The drawing under review shows one solid part. Ordinate dimensions are in mm from its lowest x, y, z. Coordinates: 2 decimals unless noted, no trailing zeros. Write each loop counter-clockwise with the first axis right and the second up, starting at its lowest first coordinate (ties: lowest second). Pieces come first, ordered by that corner, then holes.
Q1. Add section A-A, the plane x = 15. Give the boundary of the cut face in (y, z) (3 decimals), plus the area to 3 significant figures.
Q2. Add section B-B, the plane y = 0.9. Give the number of separate pieces and of enclosed holes in the cut face, plus the area to 3 significant figures.
Q3. To check wall thickness, follow probe 1 along Z at (x, y) = (25, 1.15). State the ranges of the line that lie inside material, in increasing order.
Q4. Add section D-D, the plane x = 25.5. Give the boundary of the cut face in (y, z) (3 decimals), plus the area to 3 significant figures.
Q5. Add section C-C, the plane z = 25. Give the boundary of the cut face in (x, y) (3 decimals).
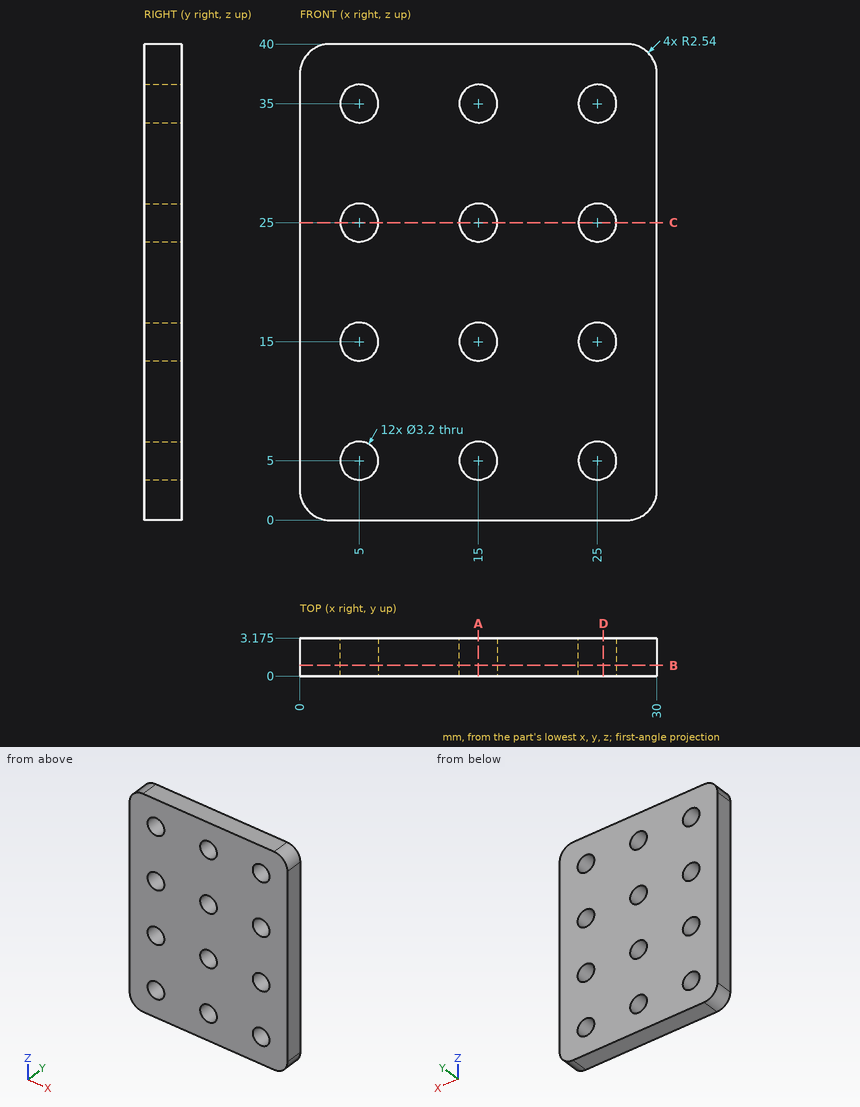
Here are the results:
1. outline: (0, 0) - (3.175, 0) - (3.175, 3.4) - (0, 3.4) - close; (0, 6.6) - (3.175, 6.6) - (3.175, 13.4) - (0, 13.4) - close; (0, 16.6) - (3.175, 16.6) - (3.175, 23.4) - (0, 23.4) - close; (0, 26.6) - (3.175, 26.6) - (3.175, 33.4) - (0, 33.4) - close; (0, 36.6) - (3.175, 36.6) - (3.175, 40) - (0, 40) - close
1. area: 86.4 mm2
2. separate pieces: 1
2. enclosed holes: 12
2. area: 1,100 mm2
3. probe 1: z = 0 to 3.4, 6.6 to 13.4, 16.6 to 23.4, 26.6 to 33.4, 36.6 to 40
4. outline: (0, 0) - (3.175, 0) - (3.175, 3.48) - (0, 3.48) - close; (0, 6.52) - (3.175, 6.52) - (3.175, 13.48) - (0, 13.48) - close; (0, 16.52) - (3.175, 16.52) - (3.175, 23.48) - (0, 23.48) - close; (0, 26.52) - (3.175, 26.52) - (3.175, 33.48) - (0, 33.48) - close; (0, 36.52) - (3.175, 36.52) - (3.175, 40) - (0, 40) - close
4. area: 88.4 mm2
5. outline: (0, 0) - (3.4, 0) - (3.4, 3.175) - (0, 3.175) - close; (6.6, 0) - (13.4, 0) - (13.4, 3.175) - (6.6, 3.175) - close; (16.6, 0) - (23.4, 0) - (23.4, 3.175) - (16.6, 3.175) - close; (26.6, 0) - (30, 0) - (30, 3.175) - (26.6, 3.175) - close
